Autodesk Inventor part; units mm, degrees
ref_plane "YZ Plane" through (0, 0, 0) normal (1, 0, 0) x (0, 1, 0)
ref_plane "XZ Plane" through (0, 0, 0) normal (0, 1, 0) x (-1, 0, 0)
ref_plane "XY Plane" through (0, 0, 0) normal (0, 0, 1) x (1, 0, 0)
sketch "Sketch2" plane through (0, 0, 0) normal (1, 0, 0) x (0, 1, 0)
  line L0 (0, 0) -> (-152.4, 0)
  line L1 (-152.4, 0) -> (-152.4, -101.6)
  line L2 (-152.4, -101.6) -> (0, -101.6)
  line L3 (0, -101.6) -> (0, 0)
  dimension "d4" = 152.4
  dimension "d5" = 101.6
extrude "Extrusion2" add sketch "Sketch2" along normal blind 5.08
sketch "Sketch4" plane through (5.08, 0, 0) normal (1, 0, 0) x (0, 0, -1)
  line L0 (0, -152.4) -> (101.6, -152.4)
  line L1 (50.8, -139.7) -> (63.5, -139.7)
  line L2 (63.5, -139.7) -> (38.1, -139.7)
  line L3 (38.1, -139.7) -> (38.1, -114.3)
  line L4 (38.1, -114.3) -> (63.5, -114.3)
  line L5 (63.5, -114.3) -> (63.5, -139.7)
  point P0 (0, 0)
  dimension "d13" = 12.7
  dimension "d14" = 25.4
  dimension "d15" = 25.4
extrude "Extrusion4" cut sketch "Sketch4" against normal blind 25.4
properties part number "Left wall"
Build history of the part. All positions in model axes, mm. A direction names the side the tool comes from. Round coordinates to 2 decimals unless told otherwise and drop trailing zeros. Loops run counter-clockwise (first coordinate to the right, second up) from the corner with the lowest first, then second, coordinate; pieces in that order, holes last. Notation, with made-up numbers: (-36.5, -36.5) -> (-15.5, -36.5) arc R32 cw to (-15.5, -7.5) -> close; hole circle Ø3 at (15.5, 58.25). An arc over 180 degrees is marked (long way). One line per item, written item: value. Start each with the question number.
Q1. Cut at B-B on x = 3.45. List the corners of the cut face in (y, z), plus the area to 3 significant figures.
Q2. 3-axis set-ups, long thin cutter, end or side, ignore diameter. For faces 1 (the face through (3, -152.4, -50)), 2 (the face through (3, -139.7, -51)): which of +Z, -Z, +X, -X, +Y, -Y reach the whole face in a straight line?
Q3. Probe line 1 along Y through (x, z) = (2.1, -49); line 2 along Z through (x, y) = (3.35, -132). List the from-to ranges inside material, lowest first.
Q4. Cut at A-A on z = -50.5. List the corners of the cut face in (x, y).
Q5. Drop flat-ended pins along their axis: pin 1 Ø2 at (x, z) = (0.5, -25.5) entering from +Y; pin 2 Ø2 at (y, z) = (-120.5, -39.5) entering from -X. Give the stop position or say it passes through.
Q6. Cut at C-C on y = -125. List the corners of the cut face in (x, z), plus the area to 3 significant figures.
Q7. Two-plate mould, pull along Z, no slides. Class faces 3 (the face through (3, -77, -101.6)), 4 (the face through (3, -75, 0)), 5 (the face through (3, -127, -38.1)): released by +Z, released by -Z, zero draft, split by the parting line, or undercut.
Computed:
1. outline: (-152.4, -101.6) -> (0, -101.6) -> (0, 0) -> (-152.4, 0) -> close; hole (-139.7, -63.5) -> (-114.3, -63.5) -> (-114.3, -38.1) -> (-139.7, -38.1) -> close
1. area: 14,800 mm²
2. face 1: +Z, -Z, +X, -X, -Y
2. face 2: +X, -X
3. line 1: -152.4 to -139.7, -114.3 to 0
3. line 2: -101.6 to -63.5, -38.1 to 0
4. outline: (0, -152.4) -> (5.08, -152.4) -> (5.08, -139.7) -> (0, -139.7) -> close; (0, -114.3) -> (5.08, -114.3) -> (5.08, 0) -> (0, 0) -> close
5. pin 1: y = 0
5. pin 2: through
6. outline: (0, -101.6) -> (5.08, -101.6) -> (5.08, -63.5) -> (0, -63.5) -> close; (0, -38.1) -> (5.08, -38.1) -> (5.08, 0) -> (0, 0) -> close
6. area: 387 mm²
7. face 3: released by -Z
7. face 4: released by +Z
7. face 5: undercut
